The drawing under review shows one solid part. Ordinate dimensions are in mm from its lowest x, y, z. Coordinates: 2 decimals unless noted, no trailing zeros. Order: outer loops, then holes, each group sorted by start corner. A loop starts at its lowest first (then second) coordinate and runs counter-clockwise, first axis right, second up. Notation, with made-up numbers: (-30.5, 79) -> (-26.5, 79) arc R28 ccw to (-26.5, 109) -> close; hole circle Ø3 at (60.25, -39). An arc over 180 degrees is marked (long way). Put each result on its own line as item: value.
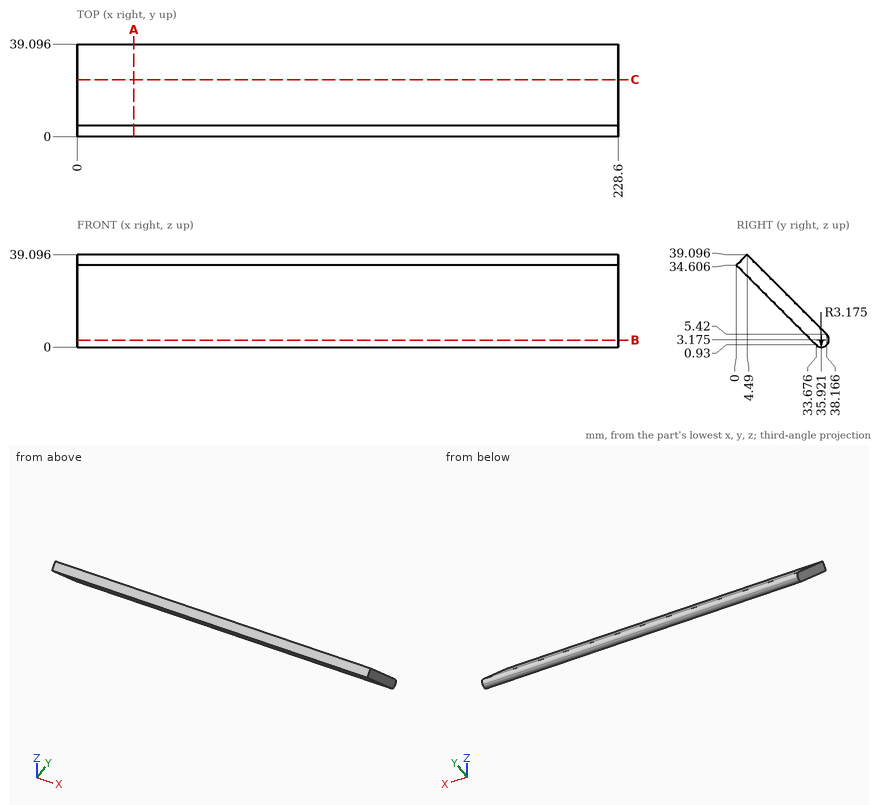
Item 1: Consider section B-B on z = 3. Write out the cut boundary in (x, y).
Answers below:
outline: (0, 31.61) -> (228.6, 31.61) -> (228.6, 39.09) -> (0, 39.09) -> close
Item 2: Consider section A-A on x = 24. Write out the cut boundary in (y, z) (3 decimals).
Answers below:
outline: (0, 34.606) -> (33.676, 0.93) arc R3.175 ccw to (38.166, 0.93) arc R3.175 ccw to (38.166, 5.42) -> (4.49, 39.096) -> close
Item 3: Consider section C-C on y = 24. Write out the cut boundary in (x, z).
Answers below:
outline: (0, 10.61) -> (228.6, 10.61) -> (228.6, 19.59) -> (0, 19.59) -> close
Item 4: For pin 1 Ø10 at (x, z) = (182.5, 13) entering from +Y; pin 2 Ø10 at (y, z) = (14, 8.5) entering from -X; pin 3 Ø4 at (x, y) = (137, 22.5) entering from -Z; pin 4 Ø3 at (x, y) = (40, 20) entering from -Z, all flat-tipped, find the tip position at first contact; note any pin that passes through.
Answers below:
pin 1: y = 35.59
pin 2: through
pin 3: z = 10.11
pin 4: z = 13.11
Item 5: For line 1 (Y direction, x = 25, z = 33); line 2 (Y direction, x = 119.5, z = 27); line 3 (Z direction, x = 140, y = 36), list the stretches that pass through material, from the lowest coordinate up. Write a range as from..to.
Answers below:
line 1: 1.61..10.59
line 2: 7.61..16.59
line 3: 0..7.59
